Geometry check sheet. Reference: the model listing, model coordinates, mm. Face numbers are marked on the shaded views. A direction names the side the tool comes from. Give positions to 0.01 mm unless a question says otherwise; leave off trailing zeros. Write each loop counter-clockwise with the first axis right and the second up, starting at its lowest first coordinate (ties: lowest second). Pieces come first, ordered by that corner, then holes. Notation, with made-up numbers: (7.25, -7) - (34.25, -7) arc R4 ccw to (34.25, 0) - close; hole circle Ø1 at (-14.75, 36). An arc over 180 degrees is marked (long way). Use a Markdown table: item, result.
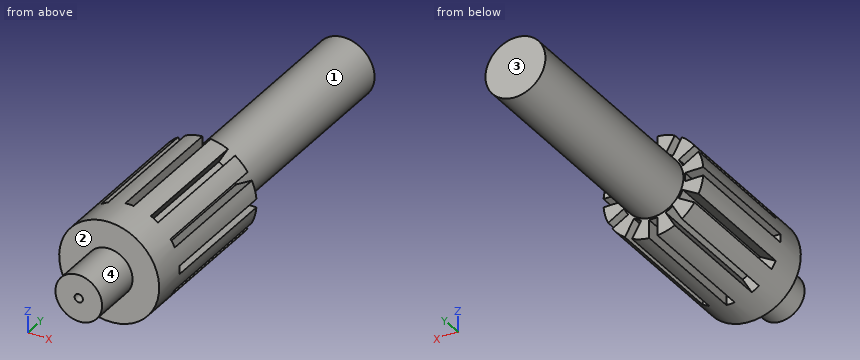
```python
from build123d import *

# Parameters (mm, degrees)
SKETCH1_R           = 15
SKETCH1_R_2         = 9
BOSS_EXTRUDE1_DEPTH = 48
SKETCH1_4_R         = 9
BOSS_EXTRUDE2_DEPTH = 68
SKETCH2_R           = 7
BOSS_EXTRUDE3_DEPTH = 15
SKETCH3_W           = 2.5
SKETCH3_H           = 6.210165372
CUT_EXTRUDE1_DEPTH  = 38
CIRPATTERN1_COUNT   = 12
SKETCH4_R           = 1.25
CUT_EXTRUDE2_DEPTH  = 15


with BuildPart() as part:
    # Sketch1 → Boss-Extrude1 (new body)
    # profile 1 of 2: a face of its own
    with BuildSketch(Plane(origin=(0, 0, 0), x_dir=(1, 0, 0), z_dir=(0, 1, 0))):
        with Locations(Location((0, 0, 0), (0, 0, 270))):
            Circle(SKETCH1_R)
        Circle(SKETCH1_R_2, mode=Mode.SUBTRACT)
    # profile 2 of 2: a face of its own
    with BuildSketch(Plane(origin=(0, 0, 0), x_dir=(1, 0, 0), z_dir=(0, 1, 0))):
        Circle(SKETCH1_R_2)
    extrude(amount=-BOSS_EXTRUDE1_DEPTH)

    # Sketch1<4> → Boss-Extrude2 (add)
    with BuildSketch(Plane(origin=(0, 0, 0), x_dir=(1, 0, 0), z_dir=(0, 1, 0))):
        with Locations(Location((0, 0, 0), (0, 0, 270))):
            Circle(SKETCH1_4_R)
    extrude(amount=BOSS_EXTRUDE2_DEPTH)

    # Sketch2 → Boss-Extrude3 (add)
    with BuildSketch(Plane.XZ.offset(48)):
        with Locations(Location((0, 0, 0), (0, 0, 270))):
            Circle(SKETCH2_R)
    extrude(amount=BOSS_EXTRUDE3_DEPTH)

    # Sketch3 → Cut-Extrude1 (cut)
    with BuildSketch(Plane(origin=(0, 0, 0), x_dir=(1, 0, 0), z_dir=(0, 1, 0))):
        with Locations((0, 12.605082686)):
            Rectangle(SKETCH3_W, SKETCH3_H)
    cut_extrude1 = extrude(amount=-CUT_EXTRUDE1_DEPTH, mode=Mode.SUBTRACT)

    # CirPattern1: Cut-Extrude1 ×12 about axis
    cirpattern1_axis = Axis((0, 0, 0), (0, 1, 0))
    for i in range(1, CIRPATTERN1_COUNT):
        add(cut_extrude1.rotate(cirpattern1_axis, i * 360 / CIRPATTERN1_COUNT), mode=Mode.SUBTRACT)

    # Sketch4 → Cut-Extrude2 (cut)
    with BuildSketch(Plane.XZ.offset(63)):
        with Locations(Location((0, 0, 0), (0, 0, 270))):
            Circle(SKETCH4_R)
    extrude(amount=-CUT_EXTRUDE2_DEPTH, mode=Mode.SUBTRACT)


solid = part.part
```
1) Mould release check, pull along Z, two halves, no side actions. Record for the marked faces 1 and 2: pulls with the +Z half, pulls with the -Z half, needs draft (parallel to the pull), parting line crosses it, or undercut.
Working result:
| item | result |
|---|---|
| face 1 | parting line crosses it |
| face 2 | needs draft |
2) Material ranges on L1, parallel to X at y = -56.5, z = 0; L2, parallel to X at y = -34, z = 9.25; L3, parallel to Y at x = 10.5, z = 3, recorded low to high. Write a range as from..to.
Working result:
| item | result |
|---|---|
| L1 | x = -7..-1.25, 1.25..7 |
| L2 | x = -11.81..-6.78, -3.9..3.9, 6.78..11.81 |
| L3 | y = -48..0 |
3) Depth check by flat-ended pin: P1, Ø3, axis at y = -26.5, z = -0.5, coming from the +X side; P2, Ø12, axis at y = 52.5, z = -12, coming from the +X side; P3, Ø0.8, axis at x = 0.5, z = -0.5, coming from the -Y side. Enter the tip coordinate at first touch or a pass-through.
Working result:
| item | result |
|---|---|
| P1 | stops at x = 14.95 |
| P2 | stops at x = 6.71 |
| P3 | stops at y = -48 |
4) Section check D-D on y = -41. Record the boundary of the cut face in (x, z).
Working result:
| item | result |
|---|---|
| outline | circle Ø30 at (0, 0) |
5) Set-up check for the marked faces 3 and 4: record each of +Z, -Z, +X, -X, +Y, -Y from which the full face is reachable in a straight line by a thin tool's end or side.
Working result:
| item | result |
|---|---|
| face 3 | +Z, -Z, +X, -X, +Y |
| face 4 | -Y |
6) Section check B-B on x = 0. Record the boundary of the cut face in (y, z), then the cut area to 3 significant figures.
Working result:
| item | result |
|---|---|
| outline | (-63, -7) - (-48, -7) - (-48, -15) - (-38, -15) - (-38, -9.5) - (0, -9.5) - (0, -9) - (68, -9) - (68, 9) - (0, 9) - (0, 9.5) - (-38, 9.5) - (-38, 15) - (-48, 15) - (-48, 7) - (-63, 7) - (-63, 1.25) - (-48, 1.25) - (-48, -1.25) - (-63, -1.25) - close |
| area | 2,420 mm² |
7) Section check A-A on z = 0. Record the boundary of the cut face in (x, y).
Working result:
| item | result |
|---|---|
| outline | (-15, -48) - (-7, -48) - (-7, -63) - (-1.25, -63) - (-1.25, -48) - (1.25, -48) - (1.25, -63) - (7, -63) - (7, -48) - (15, -48) - (15, -38) - (9.5, -38) - (9.5, 0) - (9, 0) - (9, 68) - (-9, 68) - (-9, 0) - (-9.5, 0) - (-9.5, -38) - (-15, -38) - close |
8) Section check C-C on y = 29. Record the boundary of the cut face in (x, z).
Working result:
| item | result |
|---|---|
| outline | circle Ø18 at (0, 0) |
